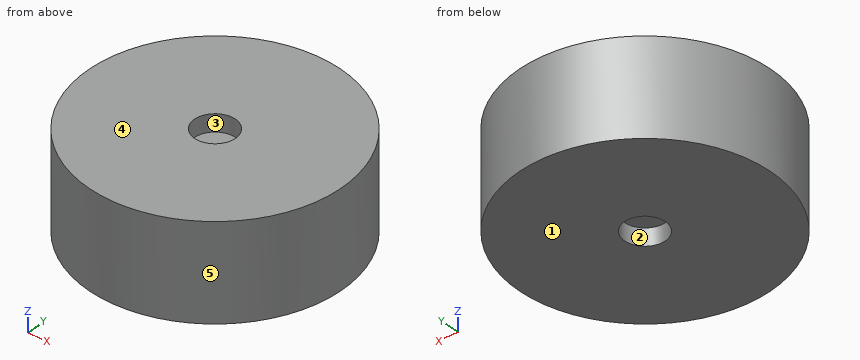
```python
from build123d import *

# Parameters (mm, degrees)
SKETCH_1_R          = 18.5
EXTRUDE_1_DEPTH     = 14
SKETCH_2_R          = 3
CUT_EXTRUDE_1_DEPTH = 2.5
SKETCH_3_R          = 3
CUT_EXTRUDE_2_DEPTH = 2.5


with BuildPart() as part:
    # 草图1 → 凸台-拉伸1 (new body)
    with BuildSketch(Plane.XY):
        Circle(SKETCH_1_R)
    extrude(amount=EXTRUDE_1_DEPTH)

    # 草图2 → 切除-拉伸1 (cut)
    with BuildSketch(Plane(origin=(0, 0, 0), x_dir=(-1, 0, 0), z_dir=(0, 0, -1))):
        Circle(SKETCH_2_R)
    extrude(amount=-CUT_EXTRUDE_1_DEPTH, mode=Mode.SUBTRACT)

    # 草图3 → 切除-拉伸2 (cut)
    with BuildSketch(Plane.XY.offset(14)):
        Circle(SKETCH_3_R)
    extrude(amount=-CUT_EXTRUDE_2_DEPTH, mode=Mode.SUBTRACT)


solid = part.part
```
CAD build for the part. Positions are in the model's coordinates, mm. Face numbers are marked on the shaded views. A direction names the side the tool comes from. Give positions to 0.01 mm unless a question says otherwise; leave off trailing zeros. Write each loop counter-clockwise with the first axis right and the second up, starting at its lowest first coordinate (ties: lowest second). Pieces come first, ordered by that corner, then holes. Notation, with made-up numbers: (65.25, 81) -> (100.25, 81) arc R35 cw to (100.25, 116) -> close; hole circle Ø11 at (46, 58.25). An arc over 180 degrees is marked (long way). Write each question's results on one line, items separated by ' | '.
1. Cut at D-D, the plane z = 8.5. Write the cut outline in (x, y), then the cut area to 3 significant figures.
Geometry check:
outline: circle Ø37 at (0, 0) | area: 1,080 mm²
2. Drop flat-ended pins along their axis: P1, Ø8, axis at x = -10.5, z = 11, coming from the -Y side; P2, Ø5, axis at y = 14, z = 6.5, coming from the -X side; P3, Ø1.5, axis at x = -7, z = 3.5, coming from the -Y side; P4, Ø6.5, axis at x = -0.5, y = 0.5, coming from the +Z side. Give the stop position or say it passes through.
Geometry check:
P1: y = -17.32 | P2: x = -14.49 | P3: y = -17.41 | P4: z = 14
3. Which spindle directions (+Z, -Z, +X, -X, +Y, -Y) get a long thin tool onto all of the face, cutting with end or side? Do the marked faces 1 and 2. Say none if no direction does.
Geometry check:
face 1: -Z, +X, -X, +Y, -Y | face 2: -Z
4. Cut at A-A, the plane y = 0. Write the cut outline in (x, z), then the cut area to 3 significant figures.
Geometry check:
outline: (-18.5, 0) -> (-3, 0) -> (-3, 2.5) -> (3, 2.5) -> (3, 0) -> (18.5, 0) -> (18.5, 14) -> (3, 14) -> (3, 11.5) -> (-3, 11.5) -> (-3, 14) -> (-18.5, 14) -> close | area: 488 mm²
5. Cut at B-B, the plane z = 12.25. Write the cut outline in (x, y), then the cut area to 3 significant figures.
Geometry check:
outline: circle Ø37 at (0, 0); hole circle Ø6 at (0, 0) | area: 1,050 mm²
6. Two-plate mould, pull along Y, no slides. Class the marked faces 3, 4 and 5: pulls with the +Y half, pulls with the -Y half, needs draft (parallel to the pull), parting line crosses it, or undercut.
Geometry check:
face 3: undercut | face 4: needs draft | face 5: parting line crosses it
7. Wall check: probe 1 along Y at (x, z) = (0, 0.75); probe 2 along X at (y, z) = (-7, 12.75); probe 3 along X at (y, z) = (-15.5, 10.5). Give the ranges that are in metal, low to high. Write a range as [from, to].
Geometry check:
probe 1: [-18.5, -3], [3, 18.5] | probe 2: [-17.12, 17.12] | probe 3: [-10.1, 10.1]
